Autodesk Inventor part; units mm, degrees
ref_plane "YZ Plane" through (0, 0, 0) normal (1, 0, 0) x (0, 1, 0)
ref_plane "XZ Plane" through (0, 0, 0) normal (0, 1, 0) x (-1, 0, 0)
ref_plane "XY Plane" through (0, 0, 0) normal (0, 0, 1) x (1, 0, 0)
sketch "Sketch1" plane through (0, 0, 0) normal (1, 0, 0) x (0, 1, 0)
  line L0 (9.4737, 39.4737) -> (-40.5263, 39.4737)
  line L1 (-40.5263, 39.4737) -> (-40.5263, -10.5263)
  line L2 (-40.5263, -10.5263) -> (9.4737, -10.5263)
  line L3 (9.4737, -10.5263) -> (9.4737, 39.4737)
  point P0 (0, 0)
  dimension "d2" = 50
  dimension "d3" = 50
extrude "Extrusion1" add sketch "Sketch1" along normal blind 70
sketch "Sketch2" plane through (70, 0, 0) normal (1, 0, 0) x (0, 0, -1)
  line L0 (-39.4737, 9.4737) -> (-39.4737, -40.5263)
  line L1 (-39.4737, -40.5263) -> (10.5263, -40.5263)
  line L2 (10.5263, 9.4737) -> (-39.4737, 9.4737)
  line L3 (10.5263, -40.5263) -> (10.5263, 9.4737)
  circle A0 centre (-14.4737, -15.5263) radius 7
  point P0 (0, 0)
  dimension "d11" = 14
extrude "Extrusion2" add sketch "Sketch2" along normal blind 190 contours A0
fillet "Fillet1" radius 15 4 edges at (35, 9.4737, 39.4737) (35, -40.5263, 39.4737) (35, 9.4737, -10.5263) (35, -40.5263, -10.5263)
sketch "Sketch3" plane through (0, -25.5263, -10.5263) normal (0, 0, -1) x (-1, 0, 0)
  line L0 (-70, 20) -> (-70, 35)
  line L1 (-70, 20) -> (0, 20)
  line L2 (0, 20) -> (0, 0)
  line L3 (0, 0) -> (-70, 0)
  line L4 (-70, 0) -> (-70, 20)
  point P0 (0, 25.5263)
extrude "Extrusion3" add sketch "Sketch3" along normal blind 7
properties part number "taladro" material "Iron, Ductile"
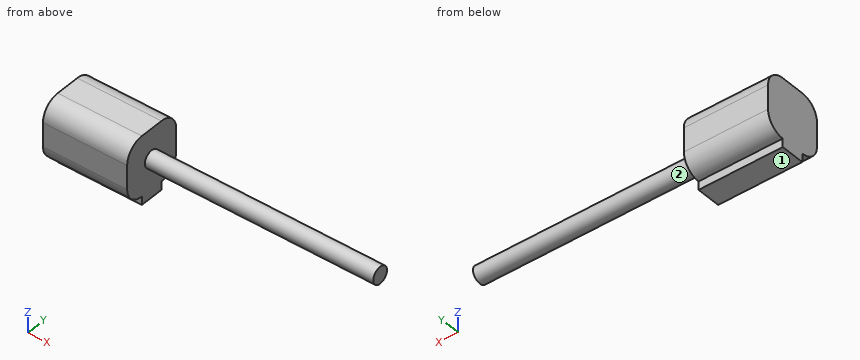
The listing builds one solid part. Answer for the finished solid, in the listing's coordinates (mm). Face numbers are marked on the shaded views. A direction names the side the tool comes from. Round coordinates to 2 decimals unless told otherwise and drop trailing zeros. Loops run counter-clockwise (first coordinate to the right, second up) from the corner with the lowest first, then second, coordinate; pieces in that order, holes last.
Q1. Section C-C, the plane y = 0.5 is taken. Determine the outline of the cut face in (x, z).
Q2. Given pin 1 Ø4 at (x, y) = (151.5, -26) entering from +Z; pin 2 Ø1 at (y, z) = (-23, 7.5) entering from -X; pin 3 Ø12 at (x, y) = (144, -5.5) entering from +Z; pin 4 Ø5 at (x, y) = (229, -12.5) entering from +Z, each flat-ended and moving along its own axis, determine where each tip first touches the part or whether it passes through.
Q3. Find the intervals of material crossed by line 1 (X direction, y = -23.5, z = 6.5); line 2 (Y direction, x = 35.5, z = -12.5); line 3 (Z direction, x = 178.5, y = -16), in increasing order.
Q4. Section A-A, the plane x = 44.5 is taken. Determine the outline of the cut face in (y, z), then the cut area to 3 significant figures.
Q5. Section B-B, the plane z = 13 is taken. Determine the outline of the cut face in (x, y), then the cut area to 3 significant figures.
Q6. Which of the six approach directions +Z, -Z, +X, -X, +Y, -Y give full straight-line access (tool end or side, diameter ignored) to the marked faces 1 and 2?
Q7. Section D-D, the plane y = -29 is taken. Determine the outline of the cut face in (x, z).
Completed:
1. outline: (0, -9.26) - (70, -9.26) - (70, 38.21) - (0, 38.21) - close
2. pin 1: passes through
2. pin 2: stops at x = 0
2. pin 3: stops at z = 20.2
2. pin 4: stops at z = 21.45
3. line 1: x = 0 to 70
3. line 2: y = -25.53 to -5.53
3. line 3: z = 7.49 to 21.46
4. outline: (-40.53, 4.47) arc R15 ccw to (-25.53, -10.53) - (-25.53, -17.53) - (-5.53, -17.53) - (-5.53, -10.53) arc R15 ccw to (9.47, 4.47) - (9.47, 24.47) arc R15 ccw to (-5.53, 39.47) - (-25.53, 39.47) arc R15 ccw to (-40.53, 24.47) - close
4. area: 2,450 mm2
5. outline: (0, -40.53) - (70, -40.53) - (70, -22.37) - (260, -22.37) - (260, -8.68) - (70, -8.68) - (70, 9.47) - (0, 9.47) - close
5. area: 6,100 mm2
6. face 1: -Z, +X, -X, +Y, -Y
6. face 2: +X
7. outline: (0, -10.12) - (70, -10.12) - (70, 39.07) - (0, 39.07) - close
